from build123d import *

# Parameters (mm, degrees)
F0_W     = 30
F0_H     = 20
F1_DEPTH = 3.75
F2_W     = 10
F2_H     = 1.875
F3_DEPTH = 24.3
F5_DEPTH = 16.12


with BuildPart() as f1:
    # F0 (on Top) → F1 (new body)
    with BuildSketch(Plane.XY):
        Rectangle(F0_W, F0_H)
    extrude(amount=F1_DEPTH)

    # F2 (on face) → F3 (cut)
    with BuildSketch(Plane.XZ.offset(10)):
        with Locations((-10, 0.9375)):
            Rectangle(F2_W, F2_H)
    extrude(amount=-F3_DEPTH, mode=Mode.SUBTRACT)

    # F4 (on face) → F5 (cut)
    with BuildSketch(Plane(origin=(0, 0, 0), x_dir=(1, 0, 0), z_dir=(0, 0, -1))):
        with BuildLine():
            ThreePointArc((1.5, -3.5), (3.974874, -2.474874), (5, 0))
            ThreePointArc((5, 0), (3.974874, 2.474874), (1.5, 3.5))
            ThreePointArc((1.5, 3.5), (-2, 0), (1.5, -3.5))
        make_face()
        with BuildLine():
            ThreePointArc((1.5, 3.5), (3.974874, 2.474874), (5, 0))
            ThreePointArc((5, 0), (6.025126, 2.474874), (8.5, 3.5))
            Line((8.5, 3.5), (1.5, 3.5))
        make_face()
        with BuildLine():
            ThreePointArc((8.5, -3.5), (6.025126, -2.474874), (5, 0))
            ThreePointArc((5, 0), (3.974874, -2.474874), (1.5, -3.5))
            Line((1.5, -3.5), (8.5, -3.5))
        make_face()
        with BuildLine():
            ThreePointArc((8.5, 3.5), (6.025126, 2.474874), (5, 0))
            ThreePointArc((5, 0), (6.025126, -2.474874), (8.5, -3.5))
            ThreePointArc((8.5, -3.5), (10.974874, -2.474874), (12, 0))
            ThreePointArc((12, 0), (10.974874, 2.474874), (8.5, 3.5))
        make_face()
    extrude(amount=-F5_DEPTH, mode=Mode.SUBTRACT)


solid = f1.part
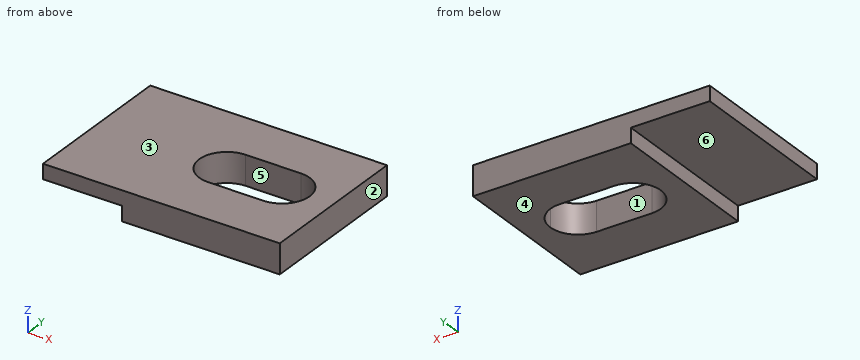
The model under review builds one solid part; all positions refer to its coordinate system, in mm. Face numbers are marked on the shaded views. A direction names the side the tool comes from. Round coordinates to 2 decimals unless told otherwise and drop trailing zeros. Loops run counter-clockwise (first coordinate to the right, second up) from the corner with the lowest first, then second, coordinate; pieces in that order, holes last. Notation, with made-up numbers: M 28,-10 L 58,-10 A31 ccw 58,29 Z; hole C 79,-20 d6. An arc over 180 degrees is marked long. Answer as CSV lines item,"result". Start each with the question number.
Item 1: Consider section C-C (y = -6.25). Write out the cut boundary in (x, z) (3 decimals).
Item 2: Insertion check: P1, Ø3, axis at x = -11.5, y = -4, coming from the -Z side (3 decimals); P2, Ø0.6, axis at y = -1, z = 0.5, coming from the -X side. Each pin has a flat end and moves straight along its axis. Give the tip position at first contact, or say it passes through.
Item 3: Consider section B-B (x = 9.25). Write out the cut boundary in (y, z).
Item 4: Wall thickness on line 1 (Y direction, x = 6, z = 3.5); line 2 (X direction, y = 4, z = 0.95); line 3 (Y direction, x = 11, z = 2.8): over which ranges is each line inside the solid? List them lowest first. Write a range as [from, to].
Item 5: Consider section D-D (z = 2.4). Write out the cut boundary in (x, y).
Item 6: Mouldability with a two-part tool opening along X and no side actions: class the marked faces 1, 2 and 3 as released by +X, released by -X, zero draft, split by the parting line, or undercut.
Item 7: Consider section A-A (z = 0.95). Write out the cut boundary in (x, y).
Item 8: For the marked faces 4, 5 and 6, list the 3-axis set-ups (+Z, -Z, +X, -X, +Y, -Y) from which the entire face can be reached by the end or side of a thin tool; tool diameter is ignored.
Answer:
1,outline,"M -15,1.875 L -5,1.875 L -5,0 L 15,0 L 15,3.75 L -15,3.75 Z"
2,P1,"stops at z = 1.875"
2,P2,"stops at x = -5"
3,outline,"M -10,0 L -3.42,0 L -3.42,3.75 L -10,3.75 Z; M 3.42,0 L 10,0 L 10,3.75 L 3.42,3.75 Z"
4,line 1,"y = [-10, -3.5], [3.5, 10]"
4,line 2,"x = [-5, 15]"
4,line 3,"y = [-10, -2.45], [2.45, 10]"
5,outline,"M -15,-10 L 15,-10 L 15,10 L -15,10 Z; hole M 1.5,-3.5 L 8.5,-3.5 A3.5 ccw 12,0 A3.5 ccw 8.5,3.5 L 1.5,3.5 A3.5 ccw Z"
6,face 1,"undercut"
6,face 2,"released by +X"
6,face 3,"zero draft"
7,outline,"M -5,-10 L 15,-10 L 15,10 L -5,10 Z; hole M 1.5,-3.5 L 8.5,-3.5 A3.5 ccw 12,0 A3.5 ccw 8.5,3.5 L 1.5,3.5 A3.5 ccw Z"
8,face 4,"-Z, +X, -X, +Y, -Y"
8,face 5,"+Z, -Z"
8,face 6,"-Z, -X, +Y, -Y"
